Autodesk Inventor part; units mm, degrees
ref_plane "YZ Plane" through (0, 0, 0) normal (1, 0, 0) x (0, 1, 0)
ref_plane "XZ Plane" through (0, 0, 0) normal (0, 1, 0) x (-1, 0, 0)
ref_plane "XY Plane" through (0, 0, 0) normal (0, 0, 1) x (1, 0, 0)
sketch "スケッチ1" plane through (0, 0, 0) normal (0, 0, 1) x (1, 0, 0)
  line L0 (0, 0) -> (4.5, 0)
  line L1 (4.5, 0) -> (4.5, 8.7)
  line L2 (4.5, 8.7) -> (0, 8.7)
  line L3 (0, 8.7) -> (0, 0)
  dimension "d0" = 4.5
  dimension "d1" = 8.7
extrude "押し出し1" add sketch "スケッチ1" against normal blind 5.6
chamfer "面取り1" distance 0.5 angle 45 1 edges at (0, 8.7, -2.8)
sketch "スケッチ2" plane through (0, 0, 0) normal (0, 0, 1) x (1, 0, 0)
  line L0 (0.4, 8.2) -> (4.1, 8.2)
  line L1 (4.1, 8.2) -> (4.1, 4.6)
  line L2 (4.1, 4.6) -> (0.4, 4.6)
  line L3 (0.4, 4.6) -> (0.4, 8.2)
  line L4 (0.4, 4.1) -> (4.1, 4.1)
  line L5 (4.1, 4.1) -> (4.1, 0.5)
  line L6 (4.1, 0.5) -> (0.4, 0.5)
  line L7 (0.4, 0.5) -> (0.4, 4.1)
  line L8 (0, 0) -> (4.5, 0)
  line L9 (4.5, 8.7) -> (0.5, 8.7)
  point P0 (2.25, 0)
  point P1 (2.25, 0.5)
  dimension "d7" = 3.7
  dimension "d8" = 3.6
  dimension "d9" = 3.6
  dimension "d10" = 0.5
  dimension "d11" = 0.5
extrude "押し出し2" cut sketch "スケッチ2" against normal blind 1.45
sketch "スケッチ3" plane through (0, 0, -1.45) normal (0, 0, 1) x (1, 0, 0)
  line L0 (4.1, 4.6) -> (0.4, 4.6)
  line L1 (4.1, 8.2) -> (4.1, 4.6)
  line L2 (0.4, 8.2) -> (4.1, 8.2)
  line L3 (0.4, 4.6) -> (0.4, 8.2)
  line L4 (4.1, 0.5) -> (0.4, 0.5)
  line L5 (4.1, 4.1) -> (4.1, 0.5)
  line L6 (0.4, 4.1) -> (4.1, 4.1)
  line L7 (0.4, 0.5) -> (0.4, 4.1)
  circle A0 centre (2.25, 6.4) radius 1.45
  circle A1 centre (2.25, 2.3) radius 1.45
  line L8 (4.1, 4.1) -> (4.1, 0.5)
  line L9 (4.1, 8.2) -> (4.1, 4.6)
  line L10 (0.4, 8.2) -> (4.1, 8.2)
  line L11 (0.4, 4.1) -> (4.1, 4.1)
  point P0 (0, 0)
  point P1 (4.1, 2.3)
  point P2 (4.1, 6.4)
  point P3 (2.25, 8.2)
  point P4 (2.25, 4.1)
  dimension "d14" = 2.9
  dimension "d15" = 2.9
extrude "押し出し3" add sketch "スケッチ3" along normal blind 1.45 contours A0 | A1
fillet "フィレット1" radius 1.45 2 edges at (0.8, 6.4, 0) (0.8, 2.3, 0)
properties part number "LBR127HLD"
Work out the finished part from the listing and answer in its coordinate system (mm). A direction names the side the tool comes from. Coordinates: 2 decimals unless noted, no trailing zeros. Order: outer loops, then holes, each group sorted by start corner. A loop starts at its lowest first (then second) coordinate and runs counter-clockwise, first axis right, second up. Notation, with made-up numbers: (77, 9.25) - (82, 9.25) arc R23 cw to (82, 20.25) - close; hole circle Ø3 at (-15.75, 64). An arc over 180 degrees is marked (long way). Put each result on its own line as item: value. Start each with the question number.
1) Find section A-A (x = 3.85). Give the vertices of the cut face in (y, z).
2) A flat-ended cylindrical pin translates along its axis: pin 1 (1.1 mm diameter, centred on x = 2, y = 3, fed in from +Z). Find the tip coordinate at first contact, or state that the pin passes through.
3) For a pull along Y with two mould halves and no side action, classify faces 3 (the flat face through (2, 0, -3)), 4 (the flat face through (4.5, 4, -3)), 5 (the flat face through (0.4, 6, -1)) as released by +Y, released by -Y, zero draft, split by the parting line, or undercut.
4) For faces 1 (the flat face through (2.2, 4.4, 0)), 2 (the flat face through (4.1, 6, -1)), determine the directions among +Z, -Z, +X, -X, +Y, -Y from which every point of the face is accessible in a straight line to the end or side of a thin tool.
5) Find the intervals of material crossed by line 1 (X direction, y = 3.5, z = -1.35); line 2 (X direction, y = 7.25, z = -0.5); line 3 (Z direction, x = 3.8, y = 2.75), in increasing order. Write a range as from..to.
6) Find section C-C (z = -0.35). State how many separate pieces and enclosed holes the cut face has, plus the area to 3 significant figures.
7) Find section B-B (y = 4.75). Give the vertices of the cut face in (x, z).
Results list:
1. outline: (0, -5.6) - (8.7, -5.6) - (8.7, 0) - (8.2, 0) - (8.2, -1.45) - (4.6, -1.45) - (4.6, 0) - (4.1, 0) - (4.1, -1.45) - (0.5, -1.45) - (0.5, 0) - (0, 0) - close
2. pin 1: stops at z = -0.01
3. face 3: released by -Y
3. face 4: zero draft
3. face 5: undercut
4. face 1: +Z, +X, -X, +Y, -Y
4. face 2: +Z
5. line 1: x = 0..0.4, 1.44..3.06, 4.1..4.5
5. line 2: x = 0..0.4, 1.56..2.94, 4.1..4.5
5. line 3: z = -5.6..-1.45
6. separate pieces: 3
6. enclosed holes: 2
6. area: 18.0 mm^2
7. outline: (0, -5.6) - (4.5, -5.6) - (4.5, 0) - (4.1, 0) - (4.1, -1.45) - (0.4, -1.45) - (0.4, 0) - (0, 0) - close
